For this review, take the finished solid that the model builds, in its own axes (mm). A direction names the side the tool comes from. Coordinates: 2 decimals unless noted, no trailing zeros. Order: outer loops, then holes, each group sorted by start corner. A loop starts at its lowest first (then second) coordinate and runs counter-clockwise, first axis right, second up. Notation, with made-up numbers: (35.5, 22.5) -> (80.5, 22.5) arc R24 ccw to (80.5, 55.5) -> close; hole circle Ø4 at (-23, 66). An arc over 180 degrees is marked (long way). Return JSON: item names as keys, results as strings. Group by question number.
Item 1: Insertion check: pin 1 (4 mm diameter, centred on y = 8, z = -74.5, fed in from -X); pin 2 (2 mm diameter, centred on x = 94.5, z = -129, fed in from -Y); pin 3 (2.5 mm diameter, centred on y = 7, z = -32.5, fed in from +X). Each pin has a flat end and moves straight along its axis. Give the tip position at first contact, or say it passes through.
Item 2: Machinability: for faces 1 (the flat face through (294, 5, -176)), 2 (the flat face through (54, 5, -176)), 3 (the flat face through (174, 5, -296)), 4 (the flat face through (173, 0, -38)), 5 (the flat face through (54, 5, -56)), which of the approach directions +Z, -Z, +X, -X, +Y, -Y give a long, thin tool a straight path to every point of the face, cutting with its end or side? Answer none if there is none.
Item 3: For line 1 along Z through (x, y) = (172, -1); line 2 along X through (y, z) = (8, -319); line 3 along Z through (x, y) = (187.5, 7.75), list the stretches that pass through material, from the lowest coordinate up.
Item 4: Take a section at B-B (z = -70). Write out the cut boundary in (x, y), then the cut area to 3 significant figures.
Item 5: Take a section at D-D (z = -247). Write out the cut boundary in (x, y), then the cut area to 3 significant figures.
Item 6: Take a section at C-C (x = 186.5). Write out the cut boundary in (y, z).
Item 7: Draft analysis for pull direction X (two halves, no side actions). For faces 6 (the flat face through (174, 5, -56)), 7 (the flat face through (0, 2, -176)), 8 (the flat face through (173, 0, -176)), state which applies: +X half, -X half, draft (parallel to the pull), parting line (faces both ways), or undercut.
Item 8: Take a section at A-A (y = -2.75). Write out the cut boundary in (x, z), then the cut area to 3 significant figures.
```python
from build123d import *

# Parameters (mm, degrees)
CROQUIS1_W              = 350
CROQUIS1_H              = 350
SALIENTE_EXTRUIR1_DEPTH = 5
CROQUIS2_W              = 350
CROQUIS2_H              = 10
SALIENTE_EXTRUIR2_DEPTH = 5
CROQUIS3_W              = 110
CROQUIS3_H              = 110
SALIENTE_EXTRUIR3_DEPTH = 5


with BuildPart() as part:
    # Croquis1 → Saliente-Extruir1 (new body)
    with BuildSketch(Plane(origin=(0, 0, 0), x_dir=(1, 0, 0), z_dir=(0, 1, 0))):
        with Locations((175, 175)):
            Rectangle(CROQUIS1_W, CROQUIS1_H)
    extrude(amount=SALIENTE_EXTRUIR1_DEPTH)

    # Croquis2 → Saliente-Extruir2 (add)
    with BuildSketch(Plane.XZ):
        with Locations((175, -5)):
            Rectangle(CROQUIS2_W, CROQUIS2_H)
        with Locations((175, -345)):
            Rectangle(CROQUIS2_W, CROQUIS2_H)
        with Locations((175, -70)):
            Rectangle(CROQUIS2_W, CROQUIS2_H)
        with Locations((175, -280)):
            Rectangle(CROQUIS2_W, CROQUIS2_H)
    extrude(amount=SALIENTE_EXTRUIR2_DEPTH)

    # Croquis3 → Saliente-Extruir3 (add)
    with BuildSketch(Plane(origin=(0, 5, 0), x_dir=(1, 0, 0), z_dir=(0, 1, 0))):
        Polygon((110, 350), (120, 350), (120, 240), (230, 240), (230, 350), (240, 350), (240, 240), (350, 240), (350, 230), (240, 230), (240, 120), (350, 120), (350, 110), (240, 110), (240, 0), (230, 0), (230, 110), (120, 110), (120, 0), (110, 0), (110, 110), (0, 110), (0, 120), (110, 120), (110, 230), (0, 230), (0, 240), (110, 240), align=None)
        with Locations((175, 175)):
            Rectangle(CROQUIS3_W, CROQUIS3_H, mode=Mode.SUBTRACT)
    extrude(amount=SALIENTE_EXTRUIR3_DEPTH)


solid = part.part
```
Findings below:
{
 "1": {"pin 1": "stops at x = 110", "pin 2": "stops at y = 0", "pin 3": "stops at x = 240"},
 "2": {"face 1": "+X, +Y", "face 2": "-X, +Y", "face 3": "-Z, +Y", "face 4": "+X, -X, -Y", "face 5": "+Z, -X, +Y"},
 "3": {"line 1": "z = -350 to -340, -285 to -275, -75 to -65, -10 to 0", "line 2": "x = 110 to 120, 230 to 240", "line 3": "z = -240 to -230, -120 to -110"},
 "4": {"outline": "(0, -5) -> (350, -5) -> (350, 5) -> (240, 5) -> (240, 10) -> (230, 10) -> (230, 5) -> (120, 5) -> (120, 10) -> (110, 10) -> (110, 5) -> (0, 5) -> close", "area": "3,600 mm2"},
 "5": {"outline": "(0, 0) -> (350, 0) -> (350, 5) -> (240, 5) -> (240, 10) -> (230, 10) -> (230, 5) -> (120, 5) -> (120, 10) -> (110, 10) -> (110, 5) -> (0, 5) -> close", "area": "1,850 mm2"},
 "6": {"outline": "(-5, -350) -> (5, -350) -> (5, -240) -> (10, -240) -> (10, -230) -> (5, -230) -> (5, -120) -> (10, -120) -> (10, -110) -> (5, -110) -> (5, 0) -> (-5, 0) -> (-5, -10) -> (0, -10) -> (0, -65) -> (-5, -65) -> (-5, -75) -> (0, -75) -> (0, -275) -> (-5, -275) -> (-5, -285) -> (0, -285) -> (0, -340) -> (-5, -340) -> close"},
 "7": {"face 6": "undercut", "face 7": "-X half", "face 8": "draft"},
 "8": {"outline": "(0, -350) -> (350, -350) -> (350, -340) -> (0, -340) -> close; (0, -285) -> (350, -285) -> (350, -275) -> (0, -275) -> close; (0, -75) -> (350, -75) -> (350, -65) -> (0, -65) -> close; (0, -10) -> (350, -10) -> (350, 0) -> (0, 0) -> close", "area": "14,000 mm2"}
}
